Geometry: final body of the model. Coordinates: model frame, mm. Give positions to 0.01 mm unless a question says otherwise; leave off trailing zeros. Write each loop counter-clockwise with the first axis right and the second up, starting at its lowest first coordinate (ties: lowest second). Pieces come first, ordered by that corner, then holes. Notation, with made-up numbers: M 53.5,-36 L 96.5,-36 A14 cw 96.5,-24 Z; hole C -14.75,32.5 d2. An arc over 180 degrees is marked long. Use a Markdown table: item, result. Add a question column.
(1) Cut plane A-A (x = 149.5). Output: boundary loops of the cut face in (y, z) (3 decimals).
(2) Pin query (flat end, axial travel): pin 1 Ø3 at (x, y) = (39, 0) entering from -Z. Return the tip coordinate at first contact, or that it passes through.
(3) Material intervals for L1, parallel to Y at x = 39, z = 2.05; L2, parallel to Y at x = 38, z = 0.9; L3, parallel to X at y = -2.5, z = 2.95, sorted ascending.
(4) Cut plane B-B (z = 2.1). State how many separate pieces and enclosed holes the cut face has, plus the area to 3 significant figures.
(5) Cut plane C-C (x = 78). Output: boundary loops of the cut face in (y, z) (3 decimals).
```python
from build123d import *

# Parameters (mm, degrees)
SKETCH_W   = 167.5
SKETCH_H   = 17
SKETCH_R   = 1.65
SKETCH_R_2 = 3.4
PAD_DEPTH  = 3.125
FILLET_R   = 5


with BuildPart() as part:
    # Sketch → Pad (new body)
    with BuildSketch(Plane.XY):
        with Locations((77.75, 0)):
            Rectangle(SKETCH_W, SKETCH_H)
        Circle(SKETCH_R, mode=Mode.SUBTRACT)
        with Locations((13, 0)):
            Circle(SKETCH_R, mode=Mode.SUBTRACT)
        with Locations((26, 0)):
            Circle(SKETCH_R, mode=Mode.SUBTRACT)
        with Locations((39, 0)):
            Circle(SKETCH_R, mode=Mode.SUBTRACT)
        with Locations((52, 0)):
            Circle(SKETCH_R, mode=Mode.SUBTRACT)
        with Locations((65, 0)):
            Circle(SKETCH_R, mode=Mode.SUBTRACT)
        with Locations((91, 0)):
            Circle(SKETCH_R, mode=Mode.SUBTRACT)
        with Locations((78, 0)):
            Circle(SKETCH_R, mode=Mode.SUBTRACT)
        with Locations((149.5, 0)):
            Circle(SKETCH_R_2, mode=Mode.SUBTRACT)
    extrude(amount=PAD_DEPTH)

    # Fillet
    fillet_edges = [part.edges().sort_by_distance(p)[0] for p in [
        (-6, -8.5, 1.5625),
        (161.5, -8.5, 1.5625),
        (161.5, 8.5, 1.5625),
        (-6, 8.5, 1.5625),
    ]]
    fillet(fillet_edges, radius=FILLET_R)


solid = part.part
```
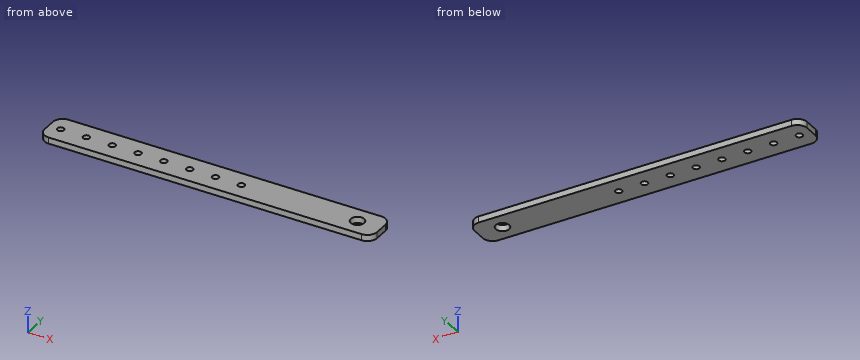
Answer list:
| question | item | result |
|---|---|---|
| 1 | outline | M -8.5,0 L -3.4,0 L -3.4,3.125 L -8.5,3.125 Z; M 3.4,0 L 8.5,0 L 8.5,3.125 L 3.4,3.125 Z |
| 2 | pin 1 | through |
| 3 | L1 | -8.5 to -1.65, 1.65 to 8.5 |
| 3 | L2 | -8.5 to -1.31, 1.31 to 8.5 |
| 3 | L3 | -6 to 147.2, 151.8 to 161.5 |
| 4 | separate pieces | 1 |
| 4 | enclosed holes | 9 |
| 4 | area | 2,720 mm² |
| 5 | outline | M -8.5,0 L -1.65,0 L -1.65,3.125 L -8.5,3.125 Z; M 1.65,0 L 8.5,0 L 8.5,3.125 L 1.65,3.125 Z |
